Verification items for the finished model (mm, model axes). A direction names the side the tool comes from. Give positions to 0.01 mm unless a question says otherwise; leave off trailing zeros. Loops run counter-clockwise (first coordinate to the right, second up) from the corner with the lowest first, then second, coordinate; pieces in that order, holes last. Notation, with made-up numbers: (48.25, 15) - (55.25, 15) arc R22 ccw to (55.25, 44) - close; hole circle Ø4 at (28.25, 82.25). An arc over 180 degrees is marked (long way). One line per item, written item: value. Start each with the question number.
1. Gauge pin test, flat ends, axial feed: pin 1 (2 mm diameter, centred on y = -37.5, z = 9, fed in from -X); pin 2 (12 mm diameter, centred on x = 149, z = 2.5, fed in from +Y) (3 decimals); pin 3 (7 mm diameter, centred on x = 38.1, y = -9.525, fed in from -Z); pin 4 (14 mm diameter, centred on x = 38.1, y = -66.675, fed in from -Z). Record the tip position at first contact, or that the pin passes through.
2. Scan lines: L1, parallel to Y at x = 38.1, z = 4.75; L2, parallel to Y at x = -188.26, z = 4.9; L3, parallel to Z at x = -31, y = -55. Record each from-to range of solid material in increasing order. Write a range as [from, to].
3. Mould release check, pull along Z, two halves, no side actions. Record for faces 6 (the flat face through (-175, -38, 13.255)), 7 (the flat face through (-170.18, -38, 3)), 8 (the flat face through (125.85, -37.567, -2.637)): pulls with the +Z half, pulls with the -Z half, needs draft (parallel to the pull), parting line crosses it, or undercut.
4. Sectioned sample at A-A (x = -38.1). Record the cut outline in (y, z).
5. Sectioned sample at B-B (x = 129). Record the cut outline in (y, z), plus the area to 3 significant figures.
6. Access from +Z, -Z, +X, -X, +Y, -Y to the whole of each face (thin tool, end or side, straight path). Record for faces 1 (the flat face through (185.26, -38, -3)), 2 (the flat face through (-1, -38, 0)), 3 (the flat face through (-125.85, -37.567, 8.987)), 4 (the flat face through (186, -38, 2.675)), 5 (the flat face through (175, -38, -1.825)).
from build123d import *

# Parameters (mm, degrees)
F0_W     = 6
F0_H     = 2.54
F0_W_2   = 63.5
F0_H_2   = 6.35
F0_W_3   = 101.6
F1_DEPTH = 76.2
F2_R     = 4.445
F2_R_2   = 1.5875
F3_DEPTH = 25.4
F4_R     = 1.5
F5_DEPTH = 13.121
F7_DEPTH = 20.161


with BuildPart() as f1:
    # F0 (on Front) → F1 (new body)
    with BuildSketch(Plane.XZ):
        Polygon((-180.18, 3.675), (-180.18, 8.175), (-170.18, 8.175), (-170.18, -1.825), (-180.18, -1.825), (-180.18, 2.675), (-185.26, 2.675), (-185.26, 0.135), (-185.26, -6.905), (-165.1, -6.905), (-165.1, 0), (-165.1, 6.35), (-165.1, 13.255), (-185.26, 13.255), (-185.26, 6.215), (-185.26, 3.675), align=None)
        with Locations((-188.26, 4.945)):
            Rectangle(F0_W, F0_H)
        with Locations((-188.26, 1.405)):
            Rectangle(F0_W, F0_H)
        Polygon((-101.6, 6.35), (-165.1, 13.255), (-165.1, 6.35), align=None)
        with Locations((-133.35, 3.175)):
            Rectangle(F0_W_2, F0_H_2)
        with Locations((-50.8, 3.175)):
            Rectangle(F0_W_3, F0_H_2)
        Polygon((-101.6, 0), (-165.1, 0), (-165.1, -6.905), align=None)
        with Locations((50.8, 3.175)):
            Rectangle(F0_W_3, F0_H_2)
        with Locations((133.35, 3.175)):
            Rectangle(F0_W_2, F0_H_2)
        Polygon((165.1, 13.255), (101.6, 6.35), (165.1, 6.35), align=None)
        Polygon((165.1, 0), (101.6, 0), (165.1, -6.905), align=None)
        Polygon((165.1, 13.255), (165.1, 6.35), (165.1, 0), (165.1, -6.905), (185.26, -6.905), (185.26, 0.135), (185.26, 2.675), (180.18, 2.675), (180.18, -1.825), (170.18, -1.825), (170.18, 8.175), (180.18, 8.175), (180.18, 3.675), (185.26, 3.675), (185.26, 6.215), (185.26, 13.255), align=None)
        with Locations((188.26, 4.945)):
            Rectangle(F0_W, F0_H)
        with Locations((188.26, 1.405)):
            Rectangle(F0_W, F0_H)
    extrude(amount=F1_DEPTH)

    # F2 (on face) → F3 (cut)
    with BuildSketch(Plane.XY.offset(6.35)):
        with Locations((-38.1, -9.525)):
            Circle(F2_R)
        with Locations((38.1, -9.525)):
            Circle(F2_R)
        with Locations((38.1, -66.675)):
            Circle(F2_R)
        with Locations((-38.1, -66.675)):
            Circle(F2_R)
        with Locations((-22.9969, -15.1031)):
            Circle(F2_R_2)
        with Locations((22.9969, -61.0969)):
            Circle(F2_R_2)
        with Locations((22.9969, -15.1031)):
            Circle(F2_R_2)
        with Locations((-22.9969, -61.0969)):
            Circle(F2_R_2)
    extrude(amount=-F3_DEPTH, mode=Mode.SUBTRACT)

    # F4 (on face) → F5 (cut, through all)
    with BuildSketch(Plane.XY.offset(6.215)):
        with Locations((-188.26, -34.1)):
            Circle(F4_R)
        with Locations((-188.26, -42.1)):
            Circle(F4_R)
        with Locations((188.26, -42.1)):
            Circle(F4_R)
        with Locations((188.26, -34.1)):
            Circle(F4_R)
    extrude(amount=-F5_DEPTH, mode=Mode.SUBTRACT)

    # F6 (on face) → F7 (cut, through all)
    with BuildSketch(Plane.XY.offset(13.255)):
        Polygon((-165.1, -19.9012937765), (-101.6, 0), (-165.1, 0), align=None)
        Polygon((-185.26, -26.2195627928), (-165.1, -19.9012937765), (-165.1, 0), (-185.26, 0), align=None)
        Polygon((-191.26, -28.1), (-185.26, -26.2195627928), (-185.26, 0), (-191.26, 0), align=None)
        Polygon((-185.26, -76.2), (-185.26, -49.9804372072), (-191.26, -48.1), (-191.26, -76.2), align=None)
        Polygon((-165.1, -76.2), (-165.1, -56.2987062235), (-185.26, -49.9804372072), (-185.26, -76.2), align=None)
        Polygon((-101.6, -76.2), (-165.1, -56.2987062235), (-165.1, -76.2), align=None)
        Polygon((191.26, -48.1), (101.6, -76.2), (191.26, -76.2), align=None)
        Polygon((191.26, 0), (101.6, 0), (191.26, -28.1), align=None)
    extrude(amount=-F7_DEPTH, mode=Mode.SUBTRACT)


solid = f1.part
Results are:
1. pin 1: stops at x = -185.26
1. pin 2: stops at y = -12.975
1. pin 3: passes through
1. pin 4: stops at z = 0
2. L1: y = [-76.2, -71.12], [-62.23, -13.97], [-5.08, 0]
2. L2: y = [-49.04, -43.6], [-40.6, -35.6], [-32.6, -27.16]
2. L3: z = [0, 6.35]
3. face 6: pulls with the +Z half
3. face 7: undercut
3. face 8: pulls with the -Z half
4. outline: (-76.2, 0) - (-71.12, 0) - (-71.12, 6.35) - (-76.2, 6.35) - close; (-62.23, 0) - (-13.97, 0) - (-13.97, 6.35) - (-62.23, 6.35) - close; (-5.08, 0) - (0, 0) - (0, 6.35) - (-5.08, 6.35) - close
5. outline: (-67.61, -2.98) - (-8.59, -2.98) - (-8.59, 9.33) - (-67.61, 9.33) - close
5. area: 727 mm^2
6. face 1: -Z, +X, +Y, -Y
6. face 2: -Z, +Y, -Y
6. face 3: +Z, +Y, -Y
6. face 4: +X, +Y, -Y
6. face 5: +Y, -Y
